```python
from build123d import *

# Parameters (mm, degrees)
BASE_DEPTH                  = 45
SKETCH2_W                   = 45
SKETCH2_H                   = 4
TOP_SKIN_DEPTH              = 62
SLIDER_BOLT_HOLE_PATTERN_D  = 6.6
DESKTOP_BOLT_HOLE_PATTERN_D = 6.7564
VISIBLE_CORNER_FILLET_R     = 10
BREAK_OTHER_CORNERS_R       = 1.5


with BuildPart() as part:
    # Sketch1 → base (new body)
    with BuildSketch(Plane.XY):
        Polygon((0, 0), (0, 100), (8, 100), (8, 4), (70, 4), (70, 0), align=None)
    extrude(amount=BASE_DEPTH)

    # Sketch2 → top skin (add)
    with BuildSketch(Plane(origin=(8, 0, 0), x_dir=(0, 0, -1), z_dir=(1, 0, 0))):
        with Locations((-22.5, 24.25)):
            Rectangle(SKETCH2_W, SKETCH2_H)
    extrude(amount=TOP_SKIN_DEPTH)

    # slider bolt hole pattern (through all)
    with Locations(Plane(origin=(8, 0, 0), x_dir=(0, 0, -1), z_dir=(1, 0, 0))):
        with Locations((-37.5, 87.5), (-7.5, 12.5), (-37.5, 12.5), (-7.5, 87.5), (-37.5, 40.5), (-7.5, 40.5)):
            Hole(SLIDER_BOLT_HOLE_PATTERN_D / 2)

    # desktop bolt hole pattern (through all)
    with Locations(Plane(origin=(0, 26.25, 0), x_dir=(1, 0, 0), z_dir=(0, 1, 0))):
        with Locations((30, -7.5), (60, -37.5), (30, -37.5), (60, -7.5)):
            Hole(DESKTOP_BOLT_HOLE_PATTERN_D / 2)

    # visible corner fillet
    visible_corner_fillet_edges = [part.edges().sort_by_distance(p)[0] for p in [
        (8, 26.25, 22.5),
    ]]
    fillet(visible_corner_fillet_edges, radius=VISIBLE_CORNER_FILLET_R)

    # break other corners
    break_other_corners_edges = [part.edges().sort_by_distance(p)[0] for p in [
        (39, 4, 45),
        (10.928932188, 29.178932188, 45),
        (10.928932188, 29.178932188, 0),
        (0, 0, 22.5),
        (0, 100, 22.5),
        (8, 100, 22.5),
        (8, 4, 22.5),
        (70, 4, 22.5),
        (70, 0, 22.5),
        (8, 13.125, 45),
        (4, 100, 45),
        (0, 50, 45),
        (70, 26.25, 22.5),
        (44, 26.25, 0),
        (70, 24.25, 0),
        (39, 22.25, 0),
        (70, 22.25, 22.5),
        (39, 22.25, 45),
        (8, 22.25, 22.5),
        (70, 24.25, 45),
        (44, 26.25, 45),
        (35, 0, 45),
        (0, 50, 0),
        (4, 100, 0),
        (8, 13.125, 0),
        (70, 2, 45),
        (39, 4, 0),
        (70, 2, 0),
        (35, 0, 0),
        (8, 68.125, 0),
        (8, 68.125, 45),
    ]]
    fillet(break_other_corners_edges, radius=BREAK_OTHER_CORNERS_R)


solid = part.part
```
Design review of the part built by this model. Coordinates are the model's own, in mm. A direction names the side the tool comes from. Give positions to 0.01 mm unless a question says otherwise; leave off trailing zeros. Write each loop counter-clockwise with the first axis right and the second up, starting at its lowest first coordinate (ties: lowest second). Pieces come first, ordered by that corner, then holes.
(1) Clearance check with flat-ended pins moving along their axes: pin 1 Ø3 at (x, z) = (60.5, 20) entering from +Y; pin 2 Ø12 at (x, z) = (31, 21.5) entering from -Y; pin 3 Ø7.5 at (y, z) = (12.5, 37.5) entering from +X; pin 4 Ø1.5 at (y, z) = (31.5, 25) entering from +X. State where each tip first meets the part, or that it passes through.
Checked values:
pin 1: stops at y = 26.25
pin 2: stops at y = 0
pin 3: stops at x = 8
pin 4: stops at x = 9.65
(2) Add section B-B (x = 30). Give the number of separate pieces and of enclosed holes in the cut face, and give its area (3 significant figures).
Checked values:
separate pieces: 6
enclosed holes: 0
area: 248 mm2
(3) Add section A-A (x = 42.5). Give the boundary of the cut face in (y, z).
Checked values:
outline: (0, 1.5) arc R1.5 ccw to (1.5, 0) - (2.5, 0) arc R1.5 ccw to (4, 1.5) - (4, 43.5) arc R1.5 ccw to (2.5, 45) - (1.5, 45) arc R1.5 ccw to (0, 43.5) - close; (22.25, 1.5) arc R1.5 ccw to (23.75, 0) - (24.75, 0) arc R1.5 ccw to (26.25, 1.5) - (26.25, 43.5) arc R1.5 ccw to (24.75, 45) - (23.75, 45) arc R1.5 ccw to (22.25, 43.5) - close
(4) Tool access review of faces 1 (the face through (8, 13, 22)), 2 (the face through (8, 68, 22)), 3 (the face through (3.94, 43.77, 7.07)): name each direction out of +Z, -Z, +X, -X, +Y, -Y from which nothing blocks a thin tool from reaching the whole face with its end or side.
Checked values:
face 1: +Z, -Z, +X
face 2: +Z, -Z, +X, +Y
face 3: +X, -X
(5) Add section C-C (y = 87.5). Give the boundary of the cut face in (x, z), and give its area (3 significant figures).
Checked values:
outline: (0, 1.5) arc R1.5 ccw to (1.5, 0) - (6.5, 0) arc R1.5 ccw to (8, 1.5) - (8, 4.2) - (0, 4.2) - close; (0, 10.8) - (8, 10.8) - (8, 34.2) - (0, 34.2) - close; (0, 40.8) - (8, 40.8) - (8, 43.5) arc R1.5 ccw to (6.5, 45) - (1.5, 45) arc R1.5 ccw to (0, 43.5) - close
area: 252 mm2
(6) Mouldability with a two-part tool opening along Z and no side actions: class faces 4 (the face through (35, 0, 22)), 5 (the face through (58.441, 24.222, 40.497)), 6 (the face through (3.94, 43.77, 37.07)), 7 (the face through (5, 50, 0)) as +Z half, -Z half, draft (parallel to the pull), parting line (faces both ways), or undercut.
Checked values:
face 4: draft
face 5: undercut
face 6: undercut
face 7: -Z half
(7) Add section D-D (z = 18). Give the boundary of the cut face in (x, y), and give its area (3 significant figures).
Checked values:
outline: (0, 1.5) arc R1.5 ccw to (1.5, 0) - (68.5, 0) arc R1.5 ccw to (70, 1.5) - (70, 2.5) arc R1.5 ccw to (68.5, 4) - (9.5, 4) arc R1.5 cw to (8, 5.5) - (8, 20.75) arc R1.5 cw to (9.5, 22.25) - (68.5, 22.25) arc R1.5 ccw to (70, 23.75) - (70, 24.75) arc R1.5 ccw to (68.5, 26.25) - (18, 26.25) arc R10 cw to (8, 36.25) - (8, 98.5) arc R1.5 ccw to (6.5, 100) - (1.5, 100) arc R1.5 ccw to (0, 98.5) - close
area: 1,320 mm2
(8) Wall thickness on line 1 along Z through (x, y) = (30, 24); line 2 along Y through (x, z) = (39.5, 40); line 3 along Y through (x, z) = (2, 37): over which ranges is each line inside the solid? List them lowest first.
Checked values:
line 1: z = 0 to 4.12, 10.88 to 34.12, 40.88 to 45
line 2: y = 0 to 4, 22.25 to 26.25
line 3: y = 0 to 9.24, 15.76 to 37.24, 43.76 to 84.24, 90.76 to 100
